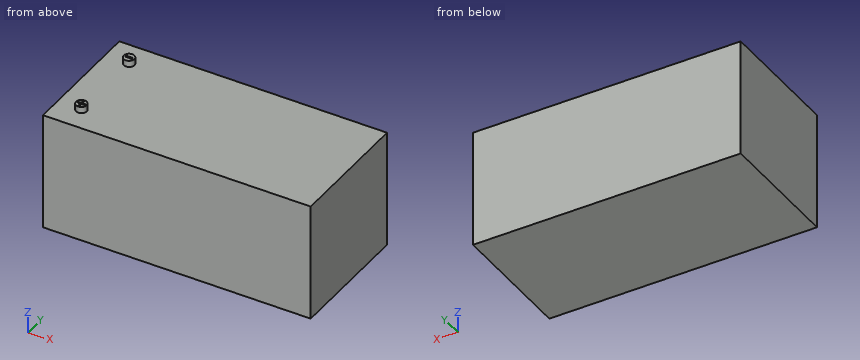
from build123d import *

# Parameters (mm, degrees)
F0_W     = 500
F0_H     = 240
F1_DEPTH = 220
F2_R     = 10
F3_DEPTH = 12
F4_W     = 12.269224124
F4_H     = 3.53
F4_W_2   = 5.75
F4_H_2   = 2.5
F4_W_3   = 2.5
F4_H_3   = 5.75
F5_DEPTH = 3


with BuildPart() as f1:
    # F0 (on Top) → F1 (new body)
    with BuildSketch(Plane.XY):
        with Locations((1.3003092026, 0)):
            Rectangle(F0_W, F0_H)
    extrude(amount=F1_DEPTH)

    # F2 (on face) → F3 (join)
    with BuildSketch(Plane.XY.offset(220)):
        with Locations((-203.6996907974, 75)):
            Circle(F2_R)
        with Locations((-203.6996907974, -75)):
            Circle(F2_R)
    extrude(amount=F3_DEPTH)

    # F4 (on face) → F5 (cut)
    with BuildSketch(Plane.XY.offset(232)):
        with Locations((-203.6996907974, 75)):
            Rectangle(F4_W, F4_H)
        with Locations((-207.8246907974, -75)):
            Rectangle(F4_W_2, F4_H_2)
        with Locations((-203.6996907974, -75)):
            Rectangle(F4_W_3, F4_H_2)
        with Locations((-199.5746907974, -75)):
            Rectangle(F4_W_2, F4_H_2)
        with Locations((-203.6996907974, -70.875)):
            Rectangle(F4_W_3, F4_H_3)
        with Locations((-203.6996907974, -79.125)):
            Rectangle(F4_W_3, F4_H_3)
    extrude(amount=-F5_DEPTH, mode=Mode.SUBTRACT)


solid = f1.part
For this review, take the finished solid that the model builds, in its own axes (mm). Give positions to 0.01 mm unless a question says otherwise; leave off trailing zeros. Loops run counter-clockwise (first coordinate to the right, second up) from the corner with the lowest first, then second, coordinate; pieces in that order, holes last. Notation, with made-up numbers: M 18.25,46 L 36.25,46 A15 cw 36.25,61 Z; hole C 73,39 d6. An arc over 180 degrees is marked long. Answer as a JSON object with one key per item and string values. Group by question number.
Q1. For probe 1 along Z at (x, y) = (-142, -38), list the stretches that pass through material, from the lowest coordinate up. Write a range as [from, to].
Q2. Add section B-B on x = -33. Give the boundary of the cut face in (y, z), and give its area (3 significant figures).
Q3. Add section A-A on y = -57.5. Give the boundary of the cut face in (x, z), and give its area (3 significant figures).
Q4. Insertion check: P1, Ø3.5, axis at y = -71, z = 231, coming from the -X side; P2, Ø2.5, axis at x = -206.5, z = 230.5, coming from the -Y side; P3, Ø0.9, axis at y = 74.5, z = 230.5, coming from the +X side. Each pin has a flat end and moves straight along its axis. Give the tip position at first contact, or say it passes through.
Checked values:
{
 "1": {"probe 1": "[0, 220]"},
 "2": {"outline": "M -120,0 L 120,0 L 120,220 L -120,220 Z", "area": "52,800 mm²"},
 "3": {"outline": "M -248.7,0 L 251.3,0 L 251.3,220 L -248.7,220 Z", "area": "110,000 mm²"},
 "4": {"P1": "x = -213.44", "P2": "y = -84.88", "P3": "x = -193.7"}
}
